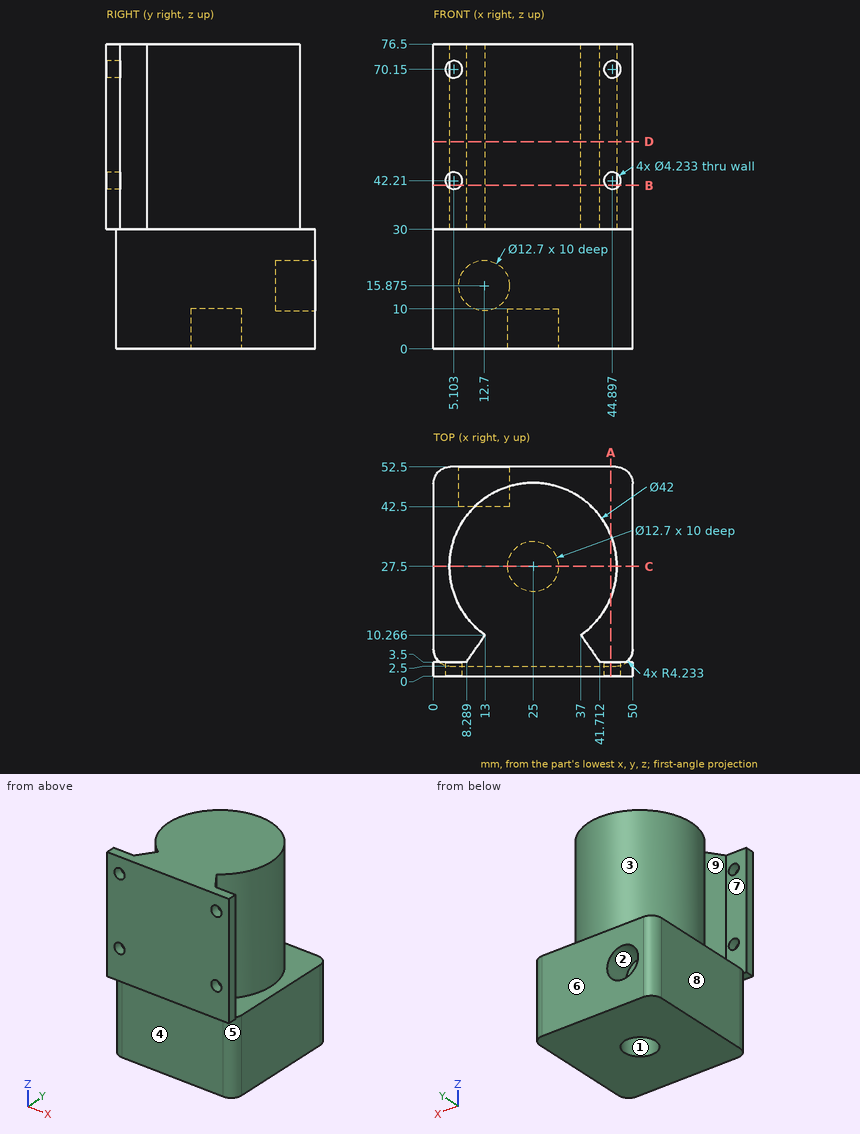
For this review, use the dimensioned drawing (mm, ordinates from the lowest corner) and the shaded views. A direction names the side the tool comes from. Round coordinates to 2 decimals unless told otherwise and drop trailing zeros. Loops run counter-clockwise (first coordinate to the right, second up) from the corner with the lowest first, then second, coordinate; pieces in that order, holes last. Notation, with made-up numbers: (61, -18.5) -> (101, -18.5) arc R21 ccw to (101, -3.5) -> close; hole circle Ø6 at (82.25, 35). An arc over 180 degrees is marked (long way). Write item = value, one per line. Start each with the question number.
Item 1: To check wall thickness, follow L1, parallel to X at y = 2, z = 42; L2, parallel to Z at x = 12.7, y = 49.25 (1 decimal); L3, parallel to Y at x = 25, z = 2. State the ranges of each line that lie inside material, in increasing order.
Item 2: Take a section at A-A on x = 44.5. Give the boundary of the cut face in (y, z) (1 decimal).
Item 3: Insertion check: pin 1 (1.5 mm diameter, centred on y = 12.5, z = 52.5, fed in from -X) (1 decimal); pin 2 (10 mm diameter, centred on x = 13.5, z = 18.5, fed in from +Y); pin 3 (4 mm diameter, centred on x = 44.9, z = 70.15, fed in from -Y); pin 4 (24 mm diameter, centred on x = 28, z = 11, fed in from -Y). Each pin has a flat end and moves straight along its axis. Give the tip position at first contact, or say it passes through.
Item 4: Take a section at B-B on z = 41. Give the boundary of the cut face in (x, y), plus the area to 3 significant figures.
Item 5: Take a section at D-D on z = 52. Give the boundary of the cut face in (x, y).
Item 6: Take a section at C-C on y = 27.5. Give the boundary of the cut face in (x, z), plus the area to 3 significant figures.
Item 7: Mouldability with a two-part tool opening along Y and no side actions: class the marked faces 6, 7, 8 and 9 as released by +Y, released by -Y, zero draft, split by the parting line, or undercut.
Item 8: For the marked faces 1, 2, 3, 4 and 5, list the 3-axis set-ups (+Z, -Z, +X, -X, +Y, -Y) from which the entire face can be reached by the end or side of a thin tool; tool diameter is ignored.
Result:
q1.L1 = 0 to 3, 7.21 to 42.79, 47 to 50
q1.L2 = 0 to 9.5, 22.2 to 30
q1.L3 = 2.5 to 21.15, 33.85 to 52.5
q2.outline = (0, 30) -> (2.5, 30) -> (2.5, 0) -> (52.5, 0) -> (52.5, 30) -> (35.3, 30) -> (35.3, 76.5) -> (19.7, 76.5) -> (19.7, 30) -> (3.5, 30) -> (3.5, 40.1) -> (0, 40.1) -> close; (0, 44.3) -> (3.5, 44.3) -> (3.5, 68.1) -> (0, 68.1) -> close; (0, 72.2) -> (3.5, 72.2) -> (3.5, 76.5) -> (0, 76.5) -> close
q3.pin_1 = 9.6
q3.pin_2 = 52.5
q3.pin_3 = 16.52
q3.pin_4 = 2.5
q4.outline = (0, 0) -> (3.37, 0) -> (3.37, 3.5) -> (0, 3.5) -> close; (6.84, 0) -> (43.16, 0) -> (43.16, 3.5) -> (41.71, 3.5) -> (37, 10.27) arc R21 ccw (long way) to (13, 10.27) -> (8.29, 3.5) -> (6.84, 3.5) -> close; (46.63, 0) -> (50, 0) -> (50, 3.5) -> (46.63, 3.5) -> close
q4.area = 1,670 mm²
q5.outline = (0, 0) -> (50, 0) -> (50, 3.5) -> (41.71, 3.5) -> (37, 10.27) arc R21 ccw (long way) to (13, 10.27) -> (8.29, 3.5) -> (0, 3.5) -> close
q6.outline = (0, 0) -> (18.65, 0) -> (18.65, 10) -> (31.35, 10) -> (31.35, 0) -> (50, 0) -> (50, 30) -> (46, 30) -> (46, 76.5) -> (4, 76.5) -> (4, 30) -> (0, 30) -> close
q6.area = 3,330 mm²
q7.face_6 = released by +Y
q7.face_7 = undercut
q7.face_8 = zero draft
q7.face_9 = undercut
q8.face_1 = -Z
q8.face_2 = +Y
q8.face_3 = +Z
q8.face_4 = -Z, +X, -X, -Y
q8.face_5 = -Z, +X, -Y
